Read the model definition and answer for the solid it produces. Units are mm, in the model's axes. A direction names the side the tool comes from. Round coordinates to 2 decimals unless told otherwise and drop trailing zeros. Order: outer loops, then holes, each group sorted by start corner. A loop starts at its lowest first (then second) coordinate and runs counter-clockwise, first axis right, second up.
from build123d import *

# Parameters (mm, degrees)
SKETCH2_W                          = 84
SKETCH2_H                          = 74
BOSS_EXTRUDE1_DEPTH                = 11
FILLET1_R                          = 18
F_8_0_8_DIAMETER_HOLE1_D           = 8
F_8_0_8_DIAMETER_HOLE1_CSINK_D     = 8.05
F_8_0_8_DIAMETER_HOLE1_CSINK_ANGLE = 90
BOSS_EXTRUDE6_DEPTH                = 4
SKETCH9_9_R                        = 23
BOSS_EXTRUDE7_DEPTH                = 17
F_8_0_28_57_DIAMETER_HOLE1_D       = 28.57
BOSS_EXTRUDE8_REACH                = 173.397
BOSS_EXTRUDE8_END_RADIUS           = 23
SKETCH18_R                         = 8.5


with BuildPart() as part:
    # Sketch2 → Boss-Extrude1 (new body)
    with BuildSketch(Plane(origin=(0, 0, 0), x_dir=(1, 0, 0), z_dir=(0, 1, 0))):
        Rectangle(SKETCH2_W, SKETCH2_H)
    extrude(amount=BOSS_EXTRUDE1_DEPTH)

    # Fillet1
    fillet1_edges = [part.edges().sort_by_distance(p)[0] for p in [
        (-42, 5.5, 37),
        (-42, 5.5, -37),
        (42, 5.5, -37),
        (42, 5.5, 37),
    ]]
    fillet(fillet1_edges, radius=FILLET1_R)

    # Ø8.0 (8) Diameter Hole1 (through all)
    with Locations(Plane(origin=(0, 11, 0), x_dir=(1, 0, 0), z_dir=(0, 1, 0))):
        with Locations((-29, 23), (29, 23), (29, -23), (-29, -23)):
            CounterSinkHole(F_8_0_8_DIAMETER_HOLE1_D / 2, F_8_0_8_DIAMETER_HOLE1_CSINK_D / 2, counter_sink_angle=F_8_0_8_DIAMETER_HOLE1_CSINK_ANGLE)

    # Sketch9 → Boss-Extrude6 (add, symmetric)
    with BuildSketch(Plane(origin=(0, 0, 0), x_dir=(0, 0, -1), z_dir=(1, 0, 0))):
        with BuildLine():
            Line((-23, 133), (-37, 11))
            Line((-37, 11), (37, 11))
            Line((37, 11), (23, 133))
            ThreePointArc((23, 133), (0, 110), (-23, 133))
        make_face()
    extrude(amount=BOSS_EXTRUDE6_DEPTH, both=True)

    # Sketch9<9> → Boss-Extrude7 (add, symmetric)
    with BuildSketch(Plane(origin=(0, 0, 0), x_dir=(0, 0, -1), z_dir=(1, 0, 0))):
        with Locations((0, 133)):
            Circle(SKETCH9_9_R)
    extrude(amount=BOSS_EXTRUDE7_DEPTH, both=True)

    # Ø8.0 (28.57) Diameter Hole1 (through all)
    with Locations(Plane(origin=(17, 0, 0), x_dir=(0, 0, -1), z_dir=(1, 0, 0))):
        with Locations((0, 133)):
            Hole(F_8_0_28_57_DIAMETER_HOLE1_D / 2)

    # Boss-Extrude8: up to this cylinder (the profile starts outside it)
    boss_extrude8_end = Plane(origin=(0, 133, 0), z_dir=(-1, 0, 0)) * Cylinder(BOSS_EXTRUDE8_END_RADIUS, 393.794, mode=Mode.PRIVATE)
    # Sketch18 → Boss-Extrude8 (add, up to the surface)
    with BuildSketch(Plane(origin=(0, 162, 0), x_dir=(-1, 0, 0), z_dir=(0, -1, 0)), mode=Mode.PRIVATE) as boss_extrude8_sk1:
        with Locations(Location((0, 0, 0), (0, 0, 270))):
            Circle(SKETCH18_R)
    boss_extrude8_tool1 = extrude(boss_extrude8_sk1.sketch, amount=BOSS_EXTRUDE8_REACH, mode=Mode.PRIVATE) - boss_extrude8_end
    add(boss_extrude8_tool1.solids().sort_by_distance((0, 162, 0))[0])


solid = part.part
Q1. Straight lines are drawn through the part: probe 1 along X at (y, z) = (3, 23); probe 2 along Y at (x, z) = (-4.5, 0) (3 decimals); probe 3 along Y at (x, z) = (-13.5, 5.5). For each, find the intervals that lie inside material, in ascending order.
Outcome:
probe 1: x = -41.55 to -33, -25 to 25, 33 to 41.55
probe 2: y = 0 to 11, 110 to 118.715, 147.285 to 162
probe 3: y = 0 to 11, 110.67 to 119.82, 146.18 to 155.33
Q2. For a pull along Y with two mould halves and no side action, classify faces 1 (the face through (-23, 11, -1)), 2 (the face through (-1, 0, -1)), 3 (the face through (-36.867, 5.577, -31.587)), 4 (the face through (0.056, 71.146, -30.098)) as released by +Y, released by -Y, zero draft, split by the parting line, or undercut.
Outcome:
face 1: undercut
face 2: released by -Y
face 3: zero draft
face 4: released by +Y
Q3. Flat-ended cylindrical pins translate along their axes: pin 1 (10 mm diameter, centred on y = 44.5, z = -1, fed in from -X); pin 2 (6 mm diameter, centred on y = 114, z = -6.5, fed in from +X); pin 3 (2 mm diameter, centred on x = -17.5, z = -18, fed in from +Y). Find the tip coordinate at first contact, or state that the pin passes through.
Outcome:
pin 1: stops at x = -4
pin 2: stops at x = 17
pin 3: stops at y = 148.34
Q4. A cutting plane is placed at D-D, the plane y = 130.5. Give the vertices of the cut face in (x, z).
Outcome:
outline: (-17, -22.86) - (-4, -22.86) - (-4, -23.29) - (4, -23.29) - (4, -22.86) - (17, -22.86) - (17, -14.06) - (-17, -14.06) - close; (-17, 14.06) - (17, 14.06) - (17, 22.86) - (4, 22.86) - (4, 23.29) - (-4, 23.29) - (-4, 22.86) - (-17, 22.86) - close
Q5. For faces 5 (the face through (17, 123, 11)), 6 (the face through (-2.55, 158.24, 8.11)), 7 (the face through (-28.479, 5.411, -26.966)), 8 (the face through (36.587, 5.577, 31.867)), 9 (the face through (23, 11, -1)), determine the directions among +Z, -Z, +X, -X, +Y, -Y from which every point of the face is accessible in a straight line to the end or side of a thin tool.
Outcome:
face 5: +Z, -Z, +X, +Y
face 6: +Y
face 7: +Y, -Y
face 8: +Z, +X, +Y, -Y
face 9: +Z, -Z, +X
Q6. A cutting plane is placed at B-B, the plane x = 11. Give the vertices of the cut face in (y, z) (3 decimals), plus the area to 3 significant figures.
Outcome:
outline: (0, -37) - (11, -37) - (11, 37) - (0, 37) - close; circle Ø46 at (133, 0); hole circle Ø28.57 at (133, 0)
area: 1,830 mm2
Q7. A cutting plane is placed at C-C, the plane x = 0. Give the vertices of the cut face in (y, z) (3 decimals).
Outcome:
outline: (0, -37) - (11, -37) - (133, -23) arc R23 ccw to (154.372, -8.5) - (162, -8.5) - (162, 8.5) - (154.372, 8.5) arc R23 ccw to (133, 23) - (11, 37) - (0, 37) - close; hole circle Ø28.57 at (133, 0)
Q8. A cutting plane is placed at A-A, the plane z = 0. Give the vertices of the cut face in (x, y) (3 decimals), plus the area to 3 significant figures.
Outcome:
outline: (-42, 0) - (42, 0) - (42, 11) - (4, 11) - (4, 110) - (17, 110) - (17, 118.715) - (-17, 118.715) - (-17, 110) - (-4, 110) - (-4, 11) - (-42, 11) - close; (-17, 147.285) - (17, 147.285) - (17, 156) - (8.5, 156) - (8.5, 162) - (-8.5, 162) - (-8.5, 156) - (-17, 156) - close
area: 2,410 mm2
